from build123d import *

# Parameters (mm, degrees)
SKETCH1_W                = 30
SKETCH1_H                = 20.75
BOSS_EXTRUDE1_DEPTH      = 4
FILLET1_R                = 1.25
SKETCH3_R                = 1.75
CUT_EXTRUDE1_DEPTH       = 10
SKETCH4_W                = 30
SKETCH4_H                = 4
BOSS_EXTRUDE2_DEPTH      = 10
FILLET2_R                = 2.5
FILLET3_R                = 2
M3_CLEARANCE_HOLE1_D     = 3.4
M3_CLEARANCE_HOLE1_DEPTH = 16
M3_CLEARANCE_HOLE1_TIP   = 1.021463052


with BuildPart() as part:
    # Sketch1 → Boss-Extrude1 (new body)
    with BuildSketch(Plane.XY):
        Rectangle(SKETCH1_W, SKETCH1_H)
    extrude(amount=BOSS_EXTRUDE1_DEPTH)

    # Fillet1
    fillet1_edges = [part.edges().sort_by_distance(p)[0] for p in [
        (-15, 10.375, 2),
        (15, 10.375, 2),
    ]]
    fillet(fillet1_edges, radius=FILLET1_R)

    # Sketch3 → Cut-Extrude1 (cut)
    with BuildSketch(Plane.XY.offset(4)):
        with Locations((-7.5, 2.375)):
            Circle(SKETCH3_R)
        with Locations((7.5, 2.375)):
            Circle(SKETCH3_R)
    extrude(amount=-CUT_EXTRUDE1_DEPTH, mode=Mode.SUBTRACT)

    # Sketch4 → Boss-Extrude2 (add)
    with BuildSketch(Plane(origin=(0, 0, 0), x_dir=(-1, 0, 0), z_dir=(0, 0, -1))):
        with Locations((0, -8.375)):
            Rectangle(SKETCH4_W, SKETCH4_H)
    extrude(amount=BOSS_EXTRUDE2_DEPTH)

    # Fillet2
    fillet2_edges = [part.edges().sort_by_distance(p)[0] for p in [
        (15, -8.375, -10),
        (-15, -8.375, -10),
    ]]
    fillet(fillet2_edges, radius=FILLET2_R)

    # Fillet3
    fillet3_edges = [part.edges().sort_by_distance(p)[0] for p in [
        (0, -6.375, 0),
    ]]
    fillet(fillet3_edges, radius=FILLET3_R)

    # M3 Clearance Hole1
    with Locations(Plane(origin=(0, -10.375, 0), x_dir=(-1, 0, 0), z_dir=(0, -1, 0))):
        with Locations((-8.75, 7), (8.75, 7)):
            Hole(M3_CLEARANCE_HOLE1_D / 2, depth=M3_CLEARANCE_HOLE1_DEPTH)
            with Locations((0, 0, -(M3_CLEARANCE_HOLE1_DEPTH + M3_CLEARANCE_HOLE1_TIP / 2))):  # 118° drill point
                Cone(0, M3_CLEARANCE_HOLE1_D / 2, M3_CLEARANCE_HOLE1_TIP, mode=Mode.SUBTRACT)


solid = part.part
CAD build for the part. Positions are in the model's coordinates, mm. A direction names the side the tool comes from. Round coordinates to 2 decimals unless told otherwise and drop trailing zeros. Write each loop counter-clockwise with the first axis right and the second up, starting at its lowest first coordinate (ties: lowest second). Pieces come first, ordered by that corner, then holes. Notation, with made-up numbers: M -11.75,-16.5 L 33.25,-16.5 A22 ccw 33.25,8.5 Z; hole C 31,-17 d3. An arc over 180 degrees is marked long. Use a Markdown table: item, result. Add a question column.
1. Slice it at A-A on z = -7. Give the cut face in (x, y) (3 decimals), then the cut area to 3 significant figures.
2. Slice it at C-C on x = 8.75. Give the cut face in (y, z) (3 decimals).
3. Pull direction X, two halves, no side cores. Call faces 1 (the face through (-14.287, -8.347, -9.248)), 2 (the face through (9.117, 1.705, 2.028)), 3 (the face through (0, 10.375, 2)): released by +X, released by -X, zero draft, split by the parting line, or undercut.
4. Slice it at D-D on y = 1.25. Give the cut face in (x, z), then the cut area to 3 significant figures.
5. 3-axis set-ups, long thin cutter, end or side, ignore diameter. For faces 4 (the face through (0, -6.375, -6)), 5 (the face through (0, 0, 4)): which of +Z, -Z, +X, -X, +Y, -Y reach the whole face in a straight line?
6. Flat gauge pins, fed straight in: P1, Ø3, axis at x = 7.5, y = 2.375, coming from the -Z side; P2, Ø4, axis at x = -4, z = -4.5, coming from the +Y side (3 decimals); P3, Ø8, axis at x = 4.5, y = 5.5, coming from the -Z side. Where does each tip first touch, or does it go through?
7. Slice it at B-B on x = -11. Give the cut face in (y, z) (3 decimals), then the cut area to 3 significant figures.
8. Drill centre lines: probe 1 along X at (y, z) = (-8.6, -7); probe 2 along Z at (x, y) = (-8.75, -9.2); probe 3 along Z at (x, y) = (-3.5, -3.5). Where is each one in solid material? Low to high.
Reply:
| question | item | result |
|---|---|---|
| 1 | outline | M -15,-10.375 L -10.45,-10.375 L -10.45,-6.375 L -15,-6.375 Z; M -7.05,-10.375 L 7.05,-10.375 L 7.05,-6.375 L -7.05,-6.375 Z; M 10.45,-10.375 L 15,-10.375 L 15,-6.375 L 10.45,-6.375 Z |
| 1 | area | 92.8 mm^2 |
| 2 | outline | M -10.375,-10 L -6.375,-10 L -6.375,-8.7 L -10.375,-8.7 Z; M -10.375,-5.3 L -6.375,-5.3 L -6.375,-2 A2 cw -4.375,0 L 1.15,0 L 1.15,4 L -10.375,4 Z; M 3.6,0 L 10.375,0 L 10.375,4 L 3.6,4 Z |
| 3 | face 1 | released by -X |
| 3 | face 2 | undercut |
| 3 | face 3 | zero draft |
| 4 | outline | M -15,0 L -8.84,0 L -8.84,4 L -15,4 Z; M -6.16,0 L 6.16,0 L 6.16,4 L -6.16,4 Z; M 8.84,0 L 15,0 L 15,4 L 8.84,4 Z |
| 4 | area | 98.6 mm^2 |
| 5 | face 4 | -Z, +X, -X, +Y |
| 5 | face 5 | +Z, +X, -X, +Y, -Y |
| 6 | P1 | passes through |
| 6 | P2 | stops at y = -6.375 |
| 6 | P3 | stops at z = 0 |
| 7 | outline | M -10.375,-10 L -6.375,-10 L -6.375,-2 A2 cw -4.375,0 L 10.375,0 L 10.375,4 L -10.375,4 Z |
| 7 | area | 124 mm^2 |
| 8 | probe 1 | x = -15 to -10.45, -7.05 to 7.05, 10.45 to 15 |
| 8 | probe 2 | z = -10 to -8.7, -5.3 to 4 |
| 8 | probe 3 | z = 0 to 4 |
